Could you check a few things on this model? Use its own coordinates, in mm. Face numbers are marked on the shaded views. A direction names the side the tool comes from. Coordinates: 2 decimals unless noted, no trailing zeros. Write each loop counter-clockwise with the first axis right and the second up, starting at its lowest first coordinate (ties: lowest second). Pieces come first, ordered by that corner, then holes.
Item 1: Thinking about a two-plate mould opening in X: for the marked faces 3, 4 and 5, which applies, +X half, -X half, draft (parallel to the pull), parting line (faces both ways), or undercut?
Item 2: For P1, Ø2, axis at y = -8, z = 3, coming from the -X side; P2, Ø8, axis at y = 9, z = 12, coming from the -X side; P3, Ø5, axis at y = 9, z = 8.5, coming from the +X side, each with a flat end and sliding along its axis, tell me the tip position at first contact or that it passes through.
Item 3: I want a section at C-C on y = 0. Please give me the cut outline in (x, z).
Item 4: I want a section at D-D on z = 3.5. Please give me the cut outline in (x, y).
Item 5: If I drill on probe 1 along Y at (x, z) = (0, 13.4); probe 2 along Y at (x, z) = (0, 17.5); probe 3 along X at (y, z) = (2.25, 13.5), over which ranges is the centre line in solid material (lowest first)?
Item 6: I want a section at B-B on x = 0. Please give me the cut outline in (y, z).
Item 7: Which directions (+Z, -Z, +X, -X, +Y, -Y) give clear straight access to the entire face, cutting with the end or side of a thin tool? Please do the marked faces 1 and 2.
Item 8: I want a section at A-A on z = 14. Please give me the cut outline in (x, y), then the cut area to 3 significant figures.
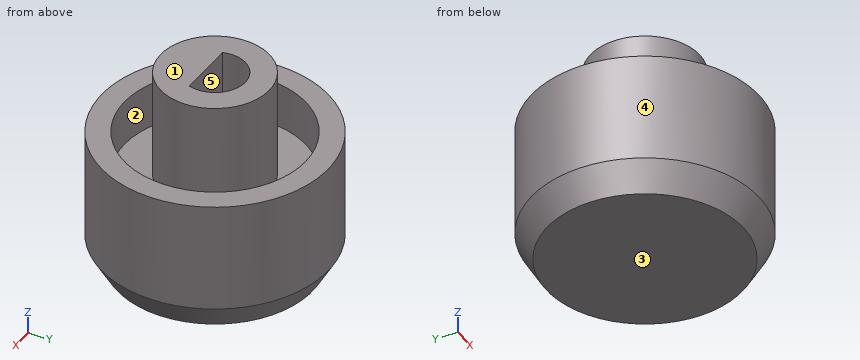
from build123d import *

# Parameters (mm, degrees)
F0_R     = 12.5
F0_R_2   = 10
F1_DEPTH = 15
F0_R_3   = 6
F2_DEPTH = 10
F3_DEPTH = 22
F4_DEPTH = 8.5
F5_SIZE2 = 1.7320508076
F5_SIZE  = 3


with BuildPart() as f1:
    # F0 (on Top) → F1 (new body)
    with BuildSketch(Plane.XY):
        Circle(F0_R)
        Circle(F0_R_2, mode=Mode.SUBTRACT)
    extrude(amount=F1_DEPTH)

    # F0 (on Top) → F2 (join)
    with BuildSketch(Plane.XY):
        Circle(F0_R_2)
        Circle(F0_R_3, mode=Mode.SUBTRACT)
    extrude(amount=F2_DEPTH)

    # F0 (on Top) → F3 (join)
    with BuildSketch(Plane.XY):
        Circle(F0_R_3)
        with BuildLine():
            ThreePointArc((-3.1972644557, -1), (0, 3.35), (3.1972644557, -1))
            Line((3.1972644557, -1), (-3.1972644557, -1))
        make_face(mode=Mode.SUBTRACT)
    extrude(amount=F3_DEPTH)

    # F0 (on Top) → F4 (join)
    with BuildSketch(Plane.XY):
        with BuildLine():
            Line((-3.1972644557, -1), (3.1972644557, -1))
            ThreePointArc((3.1972644557, -1), (0, 3.35), (-3.1972644557, -1))
        make_face()
    extrude(amount=F4_DEPTH)

    # F5
    f5_edges = [f1.edges().sort_by_distance(p)[0] for p in [
        (-12.5, 0, 0),
    ]]
    f5_side = f1.faces().sort_by_distance((-12.5, 0, 7.5))[0]
    chamfer(f5_edges, length=F5_SIZE, length2=F5_SIZE2, reference=f5_side)


solid = f1.part
Response values:
1. face 3: draft
1. face 4: parting line
1. face 5: undercut
2. P1: stops at x = -10.36
2. P2: stops at x = -11.46
2. P3: stops at x = 10.68
3. outline: (-12.5, 3) - (-10.77, 0) - (10.77, 0) - (12.5, 3) - (12.5, 15) - (10, 15) - (10, 10) - (6, 10) - (6, 22) - (3.35, 22) - (3.35, 8.5) - (-3.35, 8.5) - (-3.35, 22) - (-6, 22) - (-6, 10) - (-10, 10) - (-10, 15) - (-12.5, 15) - close
4. outline: circle Ø25 at (0, 0)
5. probe 1: y = -12.5 to -10, -6 to -1, 3.35 to 6, 10 to 12.5
5. probe 2: y = -6 to -1, 3.35 to 6
5. probe 3: x = -12.3 to -9.74, -5.56 to -2.48, 2.48 to 5.56, 9.74 to 12.3
6. outline: (-12.5, 3) - (-10.77, 0) - (10.77, 0) - (12.5, 3) - (12.5, 15) - (10, 15) - (10, 10) - (6, 10) - (6, 22) - (3.35, 22) - (3.35, 8.5) - (-1, 8.5) - (-1, 22) - (-6, 22) - (-6, 10) - (-10, 10) - (-10, 15) - (-12.5, 15) - close
7. face 1: +Z, +X, -X, +Y, -Y
7. face 2: +Z
8. outline: circle Ø25 at (0, 0); circle Ø12 at (0, 0); hole circle Ø20 at (0, 0); hole (-3.2, -1) - (3.2, -1) arc R3.35 ccw (long way) to start
8. area: 266 mm2
